from build123d import *

# Parameters (mm, degrees)
F1_DEPTH = 200
F2_W     = 158.6660303175
F2_H     = 22.1358127892
F3_DEPTH = 20
F5_DEPTH = 75
F7_R     = 5


# Not quite as in the source:
# - a feature of the source that left no trace in its solid (it failed there, or was rolled back) is left out
# - a feature names something its author has since deleted; it is built from what else it names


with BuildPart() as f1:
    # F0 (on Right) → F1 (new body)
    with BuildSketch(Plane.YZ):
        Polygon((12.9773180083, 11), (-13.0226819917, 11), (-32.7089403555, 11), (-35, -11), (35, -11), (32.6940447192, 11), align=None)
        Polygon((12.9773180083, 56), (12.9773180083, 11), (32.6940447192, 11), (27.9773180083, 56), align=None)
        Polygon((-32.7089403555, 11), (-13.0226819917, 11), (-13.0226819917, 56), (-28.0226819917, 56), align=None)
    extrude(amount=F1_DEPTH)

    # F2 (on face) → F3 (cut)
    with BuildSketch(Plane(origin=(0, 0, -11), x_dir=(1, 0, 0), z_dir=(0, 0, -1))):
        with Locations((100, 0)):
            Rectangle(F2_W, F2_H)
    extrude(amount=-F3_DEPTH, mode=Mode.SUBTRACT)

    # F4 (on Front) → F5 (cut, symmetric)
    with BuildSketch(Plane.XZ):
        Polygon((0, -11), (29.1324291224, 56), (0, 56), align=None)
        Polygon((200, -11), (200, 56), (170.8675708776, 56), align=None)
    extrude(amount=F5_DEPTH, both=True, mode=Mode.SUBTRACT)

    # F7
    f7_edges = [f1.edges().sort_by_distance(p)[0] for p in [
        (29.132429, 20.477318, 56),
        (9.565872, -0.022682, 11),
        (190.434128, -0.022682, 11),
        (14.566215, -31.511341, 22.5),
        (29.132429, -20.522682, 56),
        (19.349151, -13.022682, 33.5),
        (19.349151, 12.977318, 33.5),
        (14.566215, 31.488659, 22.5),
        (100, -13.022682, 56),
        (180.650849, -13.022682, 33.5),
        (170.867571, 20.477318, 56),
        (180.650849, 12.977318, 33.5),
        (170.867571, -20.522682, 56),
        (185.433785, -31.511341, 22.5),
        (185.433785, 31.488659, 22.5),
        (100, 12.977318, 56),
        (100, -28.022682, 56),
        (100, 27.977318, 56),
    ]]
    fillet(f7_edges, radius=F7_R)


solid = f1.part
Input: part model. Units: mm. Frame: model coordinates. A direction names the side the tool comes from. Give positions to 0.01 mm unless a question says otherwise; leave off trailing zeros. Loops run counter-clockwise (first coordinate to the right, second up) from the corner with the lowest first, then second, coordinate; pieces in that order, holes last. Notation, with made-up numbers: M 6.25,30.5 L 30.25,30.5 A11 cw 30.25,36.5 Z; hole C -25,-35 d4. An arc over 180 degrees is marked long. Use CSV: the item, a comma, the result in double quotes.
(1) Set-up query: faces 4 (the face through (19.21, -14.53, 29.61)), 5 (the face through (99, 12.977, 31)), 6 (the face through (180.51, 14.48, 30.24)). Return all of +Z, -Z, +X, -X, +Y, -Y with unobstructed straight access to the full face (end or side cutting, diameter ignored); none if empty.
Outcome:
face 4,"+Z, -X"
face 5,"+Z, +X, -X"
face 6,"+Z, +X"
(2) Pin query (flat end, axial travel): P1, Ø6, axis at x = 79.5, z = 1, coming from the +Y side; P2, Ø12, axis at x = 85, z = 31.5, coming from the +Y side; P3, Ø6, axis at y = 4.5, z = 3, coming from the -X side; P4, Ø5, axis at x = 121, y = -11, coming from the -Z side. Return the tip coordinate at first contact, or that it passes through.
Outcome:
P1,"stops at y = 34.06"
P2,"stops at y = 31.17"
P3,"stops at x = 4.78"
P4,"stops at z = -11"
(3) Section C-C, the plane y = 15.5. Return loops of the section in (x, z), plus the area to 3 significant figures.
Outcome:
outline,"M 0,-11 L 200,-11 L 191.74,7.99 A5 ccw 190.15,10 L 171.57,52.73 A4.34 ccw 167.59,55.34 L 32.41,55.34 A4.34 ccw 28.43,52.73 L 9.85,10 A5 ccw 8.26,7.99 Z"
area,"11,300 mm²"
(4) Pull-direction query (X, two-part tool) for faces 1 (the face through (100.946, 14.481, 54.574)), 2 (the face through (10.07, 0.23, 10.16)), 3 (the face through (99, 0, 9)); classes: pulls with the +X half, pulls with the -X half, needs draft (parallel to the pull), parting line crosses it, or undercut.
Outcome:
face 1,"needs draft"
face 2,"pulls with the -X half"
face 3,"undercut"
(5) Section A-A, the plane x = 81. Return loops of the section in (y, z).
Outcome:
outline,"M -35,-11 L -11.07,-11 L -11.07,9 L 11.07,9 L 11.07,-11 L 35,-11 L 28.45,51.52 A5 ccw 23.47,56 L 17.98,56 A5 ccw 12.98,51 L 12.98,11 L -13.02,11 L -13.02,51 A5 ccw -18.02,56 L -23.52,56 A5 ccw -28.49,51.52 Z"
(6) Material intervals for L1, parallel to Y at x = 177, z = 21; L2, parallel to Y at x = 23.5, z = 27.5; L3, parallel to Z at x = 17.5, y = 0, sorted ascending. Write a range as [from, to].
Outcome:
L1,"y = [-31.67, -13.02], [12.98, 31.65]"
L2,"y = [-30.99, -13.02], [12.98, 30.96]"
L3,"z = [-11, 11]"
(7) Section B-B, the plane y = 1.5. Return loops of the section in (x, z), plus the area to 3 significant figures.
Outcome:
outline,"M 0,-11 L 20.67,-11 L 20.67,9 L 179.33,9 L 179.33,-11 L 200,-11 L 191.74,7.99 A5 ccw 187.16,11 L 12.84,11 A5 ccw 8.26,7.99 Z"
area,"1,010 mm²"
